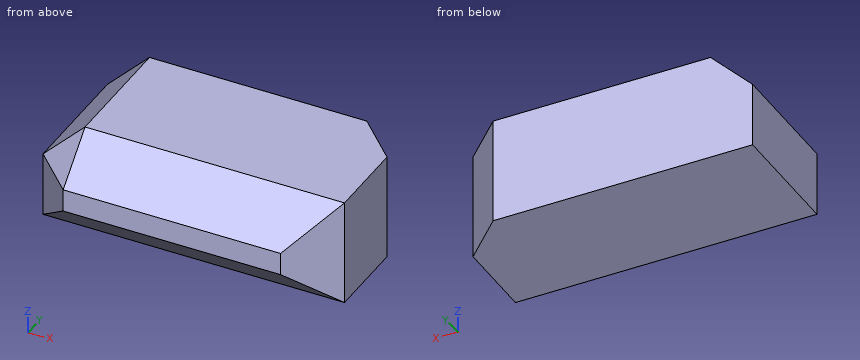
from build123d import *

# Parameters (mm, degrees)
SKETCH1_W           = 71.695166663
SKETCH1_H           = 39.401169853
BOSS_EXTRUDE1_DEPTH = 25.4
CHAMFER1_SIZE       = 10
SCALE1_SCALE        = 0.5


with BuildPart() as part:
    # Sketch1 → Boss-Extrude1 (new body)
    with BuildSketch(Plane.XY):
        with Locations((35.847583332, 19.700584926)):
            Rectangle(SKETCH1_W, SKETCH1_H)
    extrude(amount=BOSS_EXTRUDE1_DEPTH)

    # Chamfer1
    chamfer1_edges = [part.edges().sort_by_distance(p)[0] for p in [
        (0, 19.700584926, 25.4),
        (35.847583331, 0, 0),
        (71.695166663, 39.401169853, 12.7),
        (71.695166663, 0, 12.7),
        (0, 0, 12.7),
        (35.847583331, 0, 25.4),
    ]]
    chamfer(chamfer1_edges, length=CHAMFER1_SIZE)


with BuildPart() as part_1:
    # Scale1: scaled about (36.040178536, 21.517729934, 12.451063985)
    add(part.part.scale(SCALE1_SCALE).moved(Location((18.020089268, 10.758864967, 6.225531992))))


solid = part_1.part
Read the model definition and answer for the solid it produces. Units are mm, in the model's axes. Coordinates: 2 decimals unless noted, no trailing zeros. Write each loop counter-clockwise with the first axis right and the second up, starting at its lowest first coordinate (ties: lowest second). Pieces come first, ordered by that corner, then holes. Notation, with made-up numbers: M 30,44.25 L 62,44.25 A25 cw 62,66.25 Z; hole C -21,54 d6. An arc over 180 degrees is marked long. Use a Markdown table: item, result.
Q1. The part is cut by section D-D, the plane y = 27.75. Write down the section's boundary in (x, z), then the cut area to 3 significant figures.
Answer block:
| item | result |
|---|---|
| outline | M 18.02,6.23 L 51.58,6.23 L 51.58,18.93 L 23.02,18.93 L 18.02,13.93 Z |
| area | 414 mm2 |
Q2. The part is cut by section C-C, the plane x = 38.5. Write down the section's boundary in (y, z), then the cut area to 3 significant figures.
Answer block:
| item | result |
|---|---|
| outline | M 10.76,11.23 L 15.76,6.23 L 30.46,6.23 L 30.46,18.93 L 15.76,18.93 L 10.76,13.93 Z |
| area | 225 mm2 |
Q3. Each of these flat-tipped pins is pushed along its axis until it touches: pin 1 Ø1.5 at (y, z) = (26.5, 15) entering from +X; pin 2 Ø2 at (y, z) = (14, 17) entering from -X. Where does it stop, or does it pass through?
Answer block:
| item | result |
|---|---|
| pin 1 | stops at x = 53.58 |
| pin 2 | stops at x = 21.44 |
Q4. Straight lines are drawn through the part: L1, parallel to X at y = 13.25, z = 12.25; L2, parallel to X at y = 13.75, z = 11.25; L3, parallel to Y at x = 33.5, z = 14.5. For each, find the intervals that lie inside material, in ascending order. Write a range as [from, to].
Answer block:
| item | result |
|---|---|
| L1 | x = [20.53, 51.36] |
| L2 | x = [20.03, 51.86] |
| L3 | y = [11.33, 30.46] |
Q5. The part is cut by section B-B, the plane y = 16.75. Write down the section's boundary in (x, z).
Answer block:
| item | result |
|---|---|
| outline | M 18.02,6.23 L 53.87,6.23 L 53.87,18.93 L 23.02,18.93 L 18.02,13.93 Z |
Q6. The part is cut by section A-A, the plane z = 13.5. Write down the section's boundary in (x, y).
Answer block:
| item | result |
|---|---|
| outline | M 18.02,15.76 L 23.02,10.76 L 48.87,10.76 L 53.87,15.76 L 53.87,25.46 L 48.87,30.46 L 18.02,30.46 Z |
